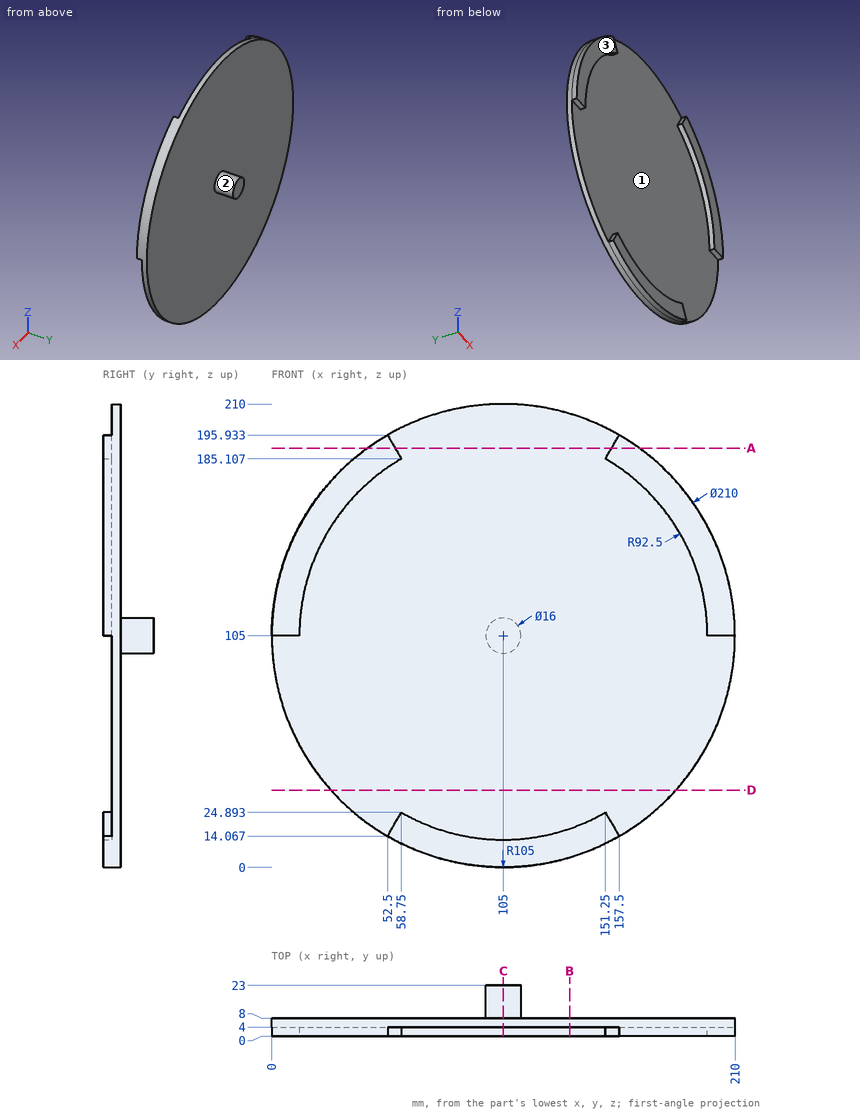
Geometry check sheet. Reference: drawing and pictorial views, mm from the part's lowest x, y, z. A direction names the side the tool comes from. Give positions to 0.01 mm unless a question says otherwise; leave off trailing zeros. Order: outer loops, then holes, each group sorted by start corner. A loop starts at its lowest first (then second) coordinate and runs counter-clockwise, first axis right, second up. Notation, with made-up numbers: (42, 3) -> (77, 3) arc R9 ccw to (77, 9) -> close; hole circle Ø2 at (54.25, 74). An arc over 180 degrees is marked (long way). Write each question's results on one line, items separated by ' | '. Start each with the question number.
(1) Sectioned sample at C-C (x = 105). Enter the section's corners in (y, z).
(2) Sectioned sample at D-D (z = 35). Enter the section's corners in (x, y), plus the area to 3 significant figures.
(3) Sectioned sample at B-B (x = 135). Enter the section's corners in (y, z).
(4) Scan lines: line 1 (Y direction, x = 186.5, z = 170.5); line 2 (Y direction, x = 146.5, z = 36); line 3 (X direction, y = 2.5, z = 129.5). Record each from-to range of solid material in increasing order.
(5) Access from +Z, -Z, +X, -X, +Y, -Y to the whole of each face (thin tool, end or side, straight path). Record for the marked faces 1, 2 and 3.
(6) Sectioned sample at A-A (z = 190). Enter the section's corners in (x, y) (1 decimal).
(7) Gauge pin test, flat ends, axial feed: P1, Ø1, axis at x = 178.5, z = 47.5, coming from the +Y side; P2, Ø10, axis at y = 3.5, z = 152.5, coming from the -X side (1 decimal); P3, Ø10, axis at y = 5.5, z = 155, coming from the +X side. Record the tip position at first contact, or that the pin passes through.
Answer below:
1) outline: (0, 0) -> (8, 0) -> (8, 97) -> (23, 97) -> (23, 113) -> (8, 113) -> (8, 210) -> (4, 210) -> (4, 12.5) -> (0, 12.5) -> close
2) outline: (26.74, 4) -> (183.26, 4) -> (183.26, 8) -> (26.74, 8) -> close | area: 626 mm2
3) outline: (0, 4.38) -> (8, 4.38) -> (8, 205.62) -> (4, 205.62) -> (4, 17.5) -> (0, 17.5) -> close
4) line 1: 0 to 8 | line 2: 4 to 8 | line 3: 2.9 to 15.8, 194.2 to 207.1
5) face 1: -Y | face 2: +Y | face 3: +Z, -Z, +X, -X, -Y
6) outline: (43.4, 0) -> (55.9, 0) -> (55.9, 4) -> (154.1, 4) -> (154.1, 0) -> (166.6, 0) -> (166.6, 8) -> (43.4, 8) -> close
7) P1: y = 8 | P2: x = 9 | P3: x = 199.87
